The drawing under review shows one solid part. Ordinate dimensions are in mm from its lowest x, y, z. A direction names the side the tool comes from. Give positions to 0.01 mm unless a question says otherwise; leave off trailing zeros. Loops run counter-clockwise (first coordinate to the right, second up) from the corner with the lowest first, then second, coordinate; pieces in that order, holes last. Notation, with made-up numbers: M 3,-8 L 25,-8 A14 cw 25,15 Z; hole C 17.5,-38 d3. An arc over 180 degrees is marked long. Put each result on its own line as item: value. Start each with the question number.
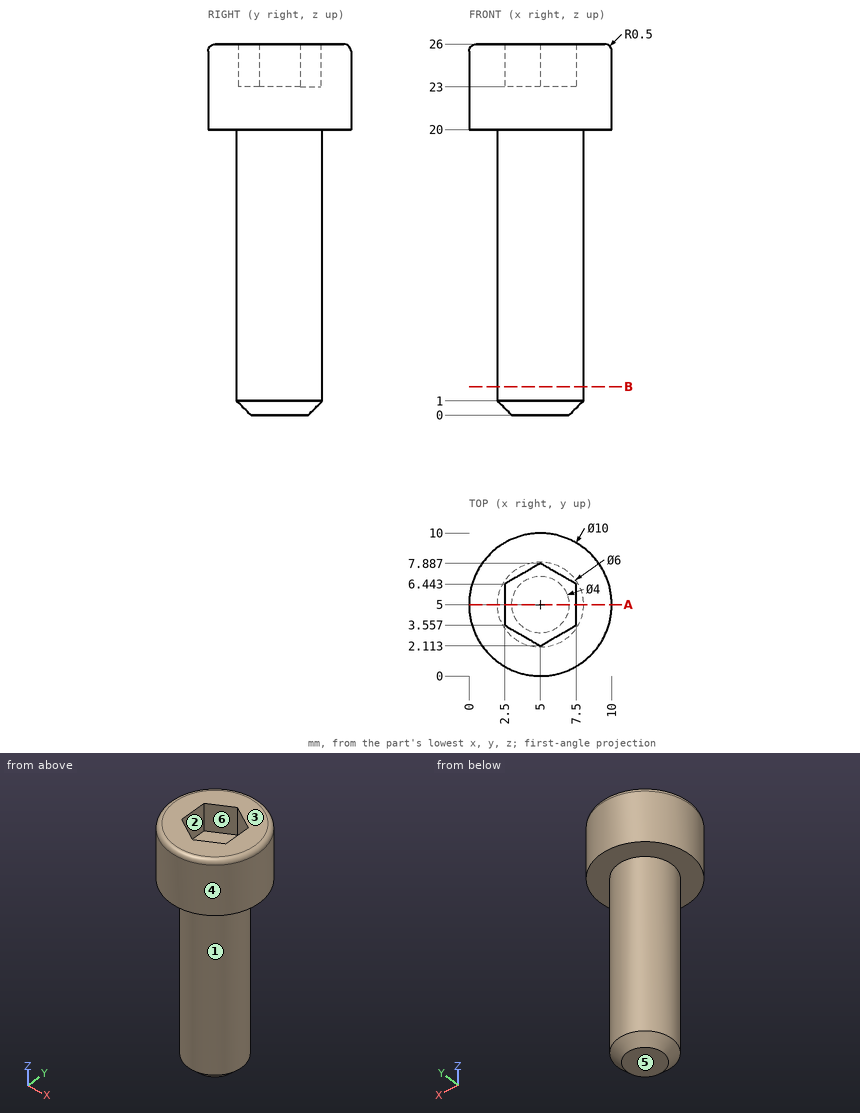
(1) We need section B-B, the plane z = 2. Write out the cut boundary in (x, y), plus the area to 3 significant figures.
(2) Insertion check: pin 1 (6 mm diameter, centred on x = 2, z = 6, fed in from -Y); pin 2 (1.4 mm diameter, centred on y = 4.5, z = 25, fed in from -X); pin 3 (1 mm diameter, centred on y = 4.5, z = 9.5, fed in from -X); pin 4 (1 mm diameter, centred on y = 2, z = 16, fed in from +X). Each pin has a flat end and moves straight along its axis. Give the tip position at first contact, or say it passes through.
(3) We need section A-A, the plane y = 5. Write out the cut boundary in (x, z).
(4) For the marked faces 1, 2 and 3, list the 3-axis set-ups (+Z, -Z, +X, -X, +Y, -Y) from which the entire face can be reached by the end or side of a thin tool; tool diameter is ignored.
(5) To check wall thickness, follow L1, parallel to X at y = 4.75, z = 24.75; L2, parallel to Z at x = 3.25, y = 8.25; L3, parallel to Y at x = 4, z = 23.5. State the ranges of each line that lie inside material, in increasing order. Write a range as [from, to].
(6) Draft analysis for pull direction X (two halves, no side actions). For the marked faces 4, 5 and 6, state which applies: +X half, -X half, draft (parallel to the pull), parting line (faces both ways), or undercut.
Check sheet entries:
1. outline: C 5,5 d6
1. area: 28.3 mm²
2. pin 1: stops at y = 2
2. pin 2: stops at x = 0
2. pin 3: stops at x = 2
2. pin 4: stops at x = 6.66
3. outline: M 0,20 L 2,20 L 2,1 L 3,0 L 7,0 L 8,1 L 8,20 L 10,20 L 10,25.5 A0.5 ccw 9.5,26 L 7.5,26 L 7.5,23 L 2.5,23 L 2.5,26 L 0.5,26 A0.5 ccw 0,25.5 Z
4. face 1: -Z
4. face 2: +Z
4. face 3: +Z, +X, -X, +Y, -Y
5. L1: x = [0.01, 2.5], [7.5, 9.99]
5. L2: z = [20, 26]
5. L3: y = [0.1, 2.69], [7.31, 9.9]
6. face 4: parting line
6. face 5: draft
6. face 6: undercut
